The listing builds one solid part. Answer for the finished solid, in the listing's coordinates (mm). Face numbers are marked on the shaded views. A direction names the side the tool comes from. Give positions to 0.01 mm unless a question says otherwise; leave off trailing zeros. Loops run counter-clockwise (first coordinate to the right, second up) from the corner with the lowest first, then second, coordinate; pieces in that order, holes last. Notation, with made-up numbers: (82, 61) - (133, 61) arc R19 cw to (133, 85) - close; hole circle Ø2 at (57, -15). An arc over 180 degrees is marked (long way). Write item = value, one per line. Start each with the question number.
1) Consider probe 1 along Z at (x, y) = (0, -4.75); probe 2 along Z at (x, y) = (-18.5, -0.5); probe 3 along X at (y, z) = (-1.5, -19). Determine where each line is inside the solid, lowest interval first.
2) The part is cut by section C-C on z = -9.5. Write down the section's boundary in (x, y), plus the area to 3 significant figures.
3) Flat-ended cylindrical pins translate along their axes: P1, Ø3, axis at y = -2.5, z = 6, coming from the +X side; P2, Ø1, axis at x = 4.5, z = 2.5, coming from the -Y side. Find the tip coordinate at first contact, or state that the pin passes through.
4) The part is cut by section A-A on x = 0. Write down the section's boundary in (y, z).
5) The mould has two halves that part along X. Classify the marked faces 1, 2, 3 and 4: +X half, -X half, draft (parallel to the pull), parting line (faces both ways), or undercut.
6) The part is cut by section B-B on z = 0. Write down the section's boundary in (x, y), plus the area to 3 significant figures.
7) Which of the six approach directions +Z, -Z, +X, -X, +Y, -Y give full straight-line access (tool end or side, diameter ignored) to the marked faces 5, 6, 7, 8 and 9?
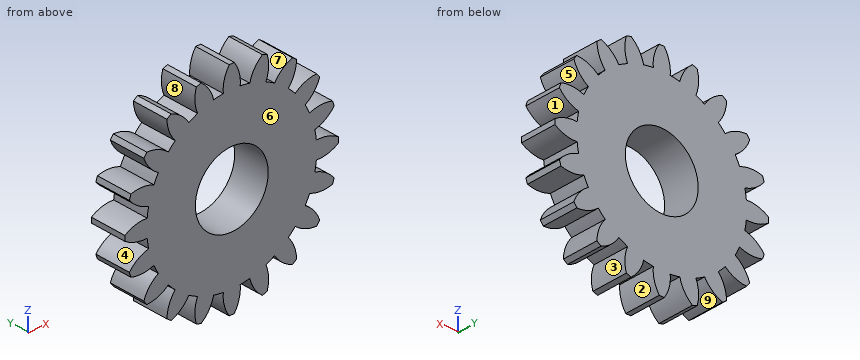
from build123d import *

# Parameters (mm, degrees)
F0_R     = 7.5
F1_DEPTH = 7.5


with BuildPart() as f1:
    # F0 (on Front) → F1 (new body)
    with BuildSketch(Plane.XZ):
        with BuildLine():
            ThreePointArc((-1.7455, 17.412732), (0, 17.5), (1.7455, 17.412732))
            ThreePointArc((1.7455, 17.412732), (1.533451, 19.81002), (0.522, 21.993806))
            Line((0.522, 21.993806), (-0.522, 21.993806))
            ThreePointArc((-0.522, 21.993806), (-1.533451, 19.81002), (-1.7455, 17.412732))
        make_face()
        with BuildLine():
            ThreePointArc((17.412732, -1.7455), (17.478169, -0.87384), (17.5, 0))
            ThreePointArc((17.5, 0), (17.478169, 0.87384), (17.412732, 1.7455))
            ThreePointArc((17.412732, 1.7455), (17.284546, 2.737603), (17.099881, 3.720761))
            ThreePointArc((17.099881, 3.720761), (16.643489, 5.407797), (16.021103, 7.040899))
            ThreePointArc((16.021103, 7.040899), (15.592614, 7.944834), (15.113175, 8.822808))
            ThreePointArc((15.113175, 8.822808), (14.157797, 10.286242), (13.061217, 11.647086))
            ThreePointArc((13.061217, 11.647086), (12.374369, 12.374369), (11.647086, 13.061217))
            ThreePointArc((11.647086, 13.061217), (10.286242, 14.157797), (8.822808, 15.113175))
            ThreePointArc((8.822808, 15.113175), (7.944834, 15.592614), (7.040899, 16.021103))
            ThreePointArc((7.040899, 16.021103), (5.407797, 16.643489), (3.720761, 17.099881))
            ThreePointArc((3.720761, 17.099881), (2.737603, 17.284546), (1.7455, 17.412732))
            ThreePointArc((1.7455, 17.412732), (0, 17.5), (-1.7455, 17.412732))
            ThreePointArc((-1.7455, 17.412732), (-2.737603, 17.284546), (-3.720761, 17.099881))
            ThreePointArc((-3.720761, 17.099881), (-5.407797, 16.643489), (-7.040899, 16.021103))
            ThreePointArc((-7.040899, 16.021103), (-7.944834, 15.592614), (-8.822808, 15.113175))
            ThreePointArc((-8.822808, 15.113175), (-10.286242, 14.157797), (-11.647086, 13.061217))
            ThreePointArc((-11.647086, 13.061217), (-12.374369, 12.374369), (-13.061217, 11.647086))
            ThreePointArc((-13.061217, 11.647086), (-14.157797, 10.286242), (-15.113175, 8.822808))
            ThreePointArc((-15.113175, 8.822808), (-15.592614, 7.944834), (-16.021103, 7.040899))
            ThreePointArc((-16.021103, 7.040899), (-16.643489, 5.407797), (-17.099881, 3.720761))
            ThreePointArc((-17.099881, 3.720761), (-17.284546, 2.737603), (-17.412732, 1.7455))
            ThreePointArc((-17.412732, 1.7455), (-17.5, 0), (-17.412732, -1.7455))
            ThreePointArc((-17.412732, -1.7455), (-17.284546, -2.737603), (-17.099881, -3.720761))
            ThreePointArc((-17.099881, -3.720761), (-16.643489, -5.407797), (-16.021103, -7.040899))
            ThreePointArc((-16.021103, -7.040899), (-15.592614, -7.944834), (-15.113175, -8.822808))
            ThreePointArc((-15.113175, -8.822808), (-14.157797, -10.286242), (-13.061217, -11.647086))
            ThreePointArc((-13.061217, -11.647086), (-12.374369, -12.374369), (-11.647086, -13.061217))
            ThreePointArc((-11.647086, -13.061217), (-10.286242, -14.157797), (-8.822808, -15.113175))
            ThreePointArc((-8.822808, -15.113175), (-7.944834, -15.592614), (-7.040899, -16.021103))
            ThreePointArc((-7.040899, -16.021103), (-5.407797, -16.643489), (-3.720761, -17.099881))
            ThreePointArc((-3.720761, -17.099881), (-2.737603, -17.284546), (-1.7455, -17.412732))
            ThreePointArc((-1.7455, -17.412732), (0, -17.5), (1.7455, -17.412732))
            ThreePointArc((1.7455, -17.412732), (2.737603, -17.284546), (3.720761, -17.099881))
            ThreePointArc((3.720761, -17.099881), (5.407797, -16.643489), (7.040899, -16.021103))
            ThreePointArc((7.040899, -16.021103), (7.944834, -15.592614), (8.822808, -15.113175))
            ThreePointArc((8.822808, -15.113175), (10.286242, -14.157797), (11.647086, -13.061217))
            ThreePointArc((11.647086, -13.061217), (12.374369, -12.374369), (13.061217, -11.647086))
            ThreePointArc((13.061217, -11.647086), (14.157797, -10.286242), (15.113175, -8.822808))
            ThreePointArc((15.113175, -8.822808), (15.592614, -7.944834), (16.021103, -7.040899))
            ThreePointArc((16.021103, -7.040899), (16.643489, -5.407797), (17.099881, -3.720761))
            ThreePointArc((17.099881, -3.720761), (17.284546, -2.737603), (17.412732, -1.7455))
        make_face()
        Circle(F0_R, mode=Mode.SUBTRACT)
        with BuildLine():
            ThreePointArc((-7.040899, 16.021103), (-5.407797, 16.643489), (-3.720761, 17.099881))
            ThreePointArc((-3.720761, 17.099881), (-4.663234, 19.314311), (-6.300008, 21.07866))
            Line((-6.300008, 21.07866), (-7.292911, 20.756046))
            ThreePointArc((-7.292911, 20.756046), (-7.580032, 18.366586), (-7.040899, 16.021103))
        make_face()
        with BuildLine():
            ThreePointArc((-11.647086, 13.061217), (-10.286242, 14.157797), (-8.822808, 15.113175))
            ThreePointArc((-8.822808, 15.113175), (-10.40345, 16.927983), (-12.505328, 18.100187))
            Line((-12.505328, 18.100187), (-13.349942, 17.486539))
            ThreePointArc((-13.349942, 17.486539), (-12.884626, 15.125303), (-11.647086, 13.061217))
        make_face()
        with BuildLine():
            ThreePointArc((-15.113175, 8.822808), (-14.157797, 10.286242), (-13.061217, 11.647086))
            ThreePointArc((-13.061217, 11.647086), (-15.125303, 12.884626), (-17.486539, 13.349942))
            Line((-17.486539, 13.349942), (-18.100187, 12.505328))
            ThreePointArc((-18.100187, 12.505328), (-16.927983, 10.40345), (-15.113175, 8.822808))
        make_face()
        with BuildLine():
            ThreePointArc((-17.099881, 3.720761), (-16.643489, 5.407797), (-16.021103, 7.040899))
            ThreePointArc((-16.021103, 7.040899), (-18.366586, 7.580032), (-20.756046, 7.292911))
            Line((-20.756046, 7.292911), (-21.07866, 6.300008))
            ThreePointArc((-21.07866, 6.300008), (-19.314311, 4.663234), (-17.099881, 3.720761))
        make_face()
        with BuildLine():
            ThreePointArc((-17.412732, -1.7455), (-17.5, 0), (-17.412732, 1.7455))
            ThreePointArc((-17.412732, 1.7455), (-19.81002, 1.533451), (-21.993806, 0.522))
            Line((-21.993806, 0.522), (-21.993806, -0.522))
            ThreePointArc((-21.993806, -0.522), (-19.81002, -1.533451), (-17.412732, -1.7455))
        make_face()
        with BuildLine():
            ThreePointArc((-20.756046, -7.292911), (-18.366586, -7.580032), (-16.021103, -7.040899))
            ThreePointArc((-16.021103, -7.040899), (-16.643489, -5.407797), (-17.099881, -3.720761))
            ThreePointArc((-17.099881, -3.720761), (-19.314311, -4.663234), (-21.07866, -6.300008))
            Line((-21.07866, -6.300008), (-20.756046, -7.292911))
        make_face()
        with BuildLine():
            ThreePointArc((-17.486539, -13.349942), (-15.125303, -12.884626), (-13.061217, -11.647086))
            ThreePointArc((-13.061217, -11.647086), (-14.157797, -10.286242), (-15.113175, -8.822808))
            ThreePointArc((-15.113175, -8.822808), (-16.927983, -10.40345), (-18.100187, -12.505328))
            Line((-18.100187, -12.505328), (-17.486539, -13.349942))
        make_face()
        with BuildLine():
            ThreePointArc((-12.505328, -18.100187), (-10.40345, -16.927983), (-8.822808, -15.113175))
            ThreePointArc((-8.822808, -15.113175), (-10.286242, -14.157797), (-11.647086, -13.061217))
            ThreePointArc((-11.647086, -13.061217), (-12.884626, -15.125303), (-13.349942, -17.486539))
            Line((-13.349942, -17.486539), (-12.505328, -18.100187))
        make_face()
        with BuildLine():
            ThreePointArc((-6.300008, -21.07866), (-4.663234, -19.314311), (-3.720761, -17.099881))
            ThreePointArc((-3.720761, -17.099881), (-5.407797, -16.643489), (-7.040899, -16.021103))
            ThreePointArc((-7.040899, -16.021103), (-7.580032, -18.366586), (-7.292911, -20.756046))
            Line((-7.292911, -20.756046), (-6.300008, -21.07866))
        make_face()
        with BuildLine():
            ThreePointArc((0.522, -21.993806), (1.533451, -19.81002), (1.7455, -17.412732))
            ThreePointArc((1.7455, -17.412732), (0, -17.5), (-1.7455, -17.412732))
            ThreePointArc((-1.7455, -17.412732), (-1.533451, -19.81002), (-0.522, -21.993806))
            Line((-0.522, -21.993806), (0.522, -21.993806))
        make_face()
        with BuildLine():
            ThreePointArc((7.292911, -20.756046), (7.580032, -18.366586), (7.040899, -16.021103))
            ThreePointArc((7.040899, -16.021103), (5.407797, -16.643489), (3.720761, -17.099881))
            ThreePointArc((3.720761, -17.099881), (4.663234, -19.314311), (6.300008, -21.07866))
            Line((6.300008, -21.07866), (7.292911, -20.756046))
        make_face()
        with BuildLine():
            ThreePointArc((13.349942, -17.486539), (12.884626, -15.125303), (11.647086, -13.061217))
            ThreePointArc((11.647086, -13.061217), (10.286242, -14.157797), (8.822808, -15.113175))
            ThreePointArc((8.822808, -15.113175), (10.40345, -16.927983), (12.505328, -18.100187))
            Line((12.505328, -18.100187), (13.349942, -17.486539))
        make_face()
        with BuildLine():
            ThreePointArc((21.07866, -6.300008), (19.314311, -4.663234), (17.099881, -3.720761))
            ThreePointArc((17.099881, -3.720761), (16.643489, -5.407797), (16.021103, -7.040899))
            ThreePointArc((16.021103, -7.040899), (18.366586, -7.580032), (20.756046, -7.292911))
            Line((20.756046, -7.292911), (21.07866, -6.300008))
        make_face()
        with BuildLine():
            ThreePointArc((17.412732, 1.7455), (17.478169, 0.87384), (17.5, 0))
            ThreePointArc((17.5, 0), (17.478169, -0.87384), (17.412732, -1.7455))
            ThreePointArc((17.412732, -1.7455), (19.81002, -1.533451), (21.993806, -0.522))
            Line((21.993806, -0.522), (21.993806, 0.522))
            ThreePointArc((21.993806, 0.522), (19.81002, 1.533451), (17.412732, 1.7455))
        make_face()
        with BuildLine():
            ThreePointArc((18.100187, -12.505328), (16.927983, -10.40345), (15.113175, -8.822808))
            ThreePointArc((15.113175, -8.822808), (14.157797, -10.286242), (13.061217, -11.647086))
            ThreePointArc((13.061217, -11.647086), (15.125303, -12.884626), (17.486539, -13.349942))
            Line((17.486539, -13.349942), (18.100187, -12.505328))
        make_face()
        with BuildLine():
            ThreePointArc((16.021103, 7.040899), (16.643489, 5.407797), (17.099881, 3.720761))
            ThreePointArc((17.099881, 3.720761), (19.314311, 4.663234), (21.07866, 6.300008))
            Line((21.07866, 6.300008), (20.756046, 7.292911))
            ThreePointArc((20.756046, 7.292911), (18.366586, 7.580032), (16.021103, 7.040899))
        make_face()
        with BuildLine():
            ThreePointArc((13.061217, 11.647086), (14.157797, 10.286242), (15.113175, 8.822808))
            ThreePointArc((15.113175, 8.822808), (16.927983, 10.40345), (18.100187, 12.505328))
            Line((18.100187, 12.505328), (17.486539, 13.349942))
            ThreePointArc((17.486539, 13.349942), (15.125303, 12.884626), (13.061217, 11.647086))
        make_face()
        with BuildLine():
            ThreePointArc((8.822808, 15.113175), (10.286242, 14.157797), (11.647086, 13.061217))
            ThreePointArc((11.647086, 13.061217), (12.884626, 15.125303), (13.349942, 17.486539))
            Line((13.349942, 17.486539), (12.505328, 18.100187))
            ThreePointArc((12.505328, 18.100187), (10.40345, 16.927983), (8.822808, 15.113175))
        make_face()
        with BuildLine():
            ThreePointArc((3.720761, 17.099881), (5.407797, 16.643489), (7.040899, 16.021103))
            ThreePointArc((7.040899, 16.021103), (7.580032, 18.366586), (7.292911, 20.756046))
            Line((7.292911, 20.756046), (6.300008, 21.07866))
            ThreePointArc((6.300008, 21.07866), (4.663234, 19.314311), (3.720761, 17.099881))
        make_face()
    extrude(amount=F1_DEPTH)


solid = f1.part
Answer below:
q1.probe_1 = -21.99 to -7.5, 7.5 to 21.99
q1.probe_2 = -7.59 to -4.21, -1.75 to 1.75, 4.21 to 7.59
q1.probe_3 = -7.59 to -4.47, -1.7 to 1.7, 4.47 to 7.59
q2.outline = (-16.05, -7.5) - (16.05, -7.5) - (16.05, 0) - (-16.05, 0) - close
q2.area = 241 mm2
q3.P1 = 21.08
q3.P2 = through
q4.outline = (-7.5, -21.99) - (0, -21.99) - (0, -7.5) - (-7.5, -7.5) - close; (-7.5, 7.5) - (0, 7.5) - (0, 21.99) - (-7.5, 21.99) - close
q5.face_1 = +X half
q5.face_2 = undercut
q5.face_3 = undercut
q5.face_4 = -X half
q6.outline = (-21.99, -7.5) - (-7.5, -7.5) - (-7.5, 0) - (-21.99, 0) - close; (7.5, -7.5) - (21.99, -7.5) - (21.99, 0) - (7.5, 0) - close
q6.area = 217 mm2
q7.face_5 = +X, +Y, -Y
q7.face_6 = +Z, -Z, +X, -X, -Y
q7.face_7 = +Z, +Y, -Y
q7.face_8 = +Y, -Y
q7.face_9 = -Z, +Y, -Y
